Build history of the part. All positions in model axes, mm. Face numbers are marked on the shaded views. A direction names the side the tool comes from. Give positions to 0.01 mm unless a question says otherwise; leave off trailing zeros. Order: outer loops, then holes, each group sorted by start corner. A loop starts at its lowest first (then second) coordinate and runs counter-clockwise, first axis right, second up. Notation, with made-up numbers: (41, 30) -> (47, 30) arc R27 ccw to (47, 64) -> close; hole circle Ø4 at (-7.5, -34). An arc over 180 degrees is marked (long way). One line per item, written item: value. Start each with the question number.
(1) Probe line 1 (Y direction, x = -20.5, z = 8.5); line 2 (Z direction, x = -11, y = 18.5); line 3 (Y direction, x = 6.5, z = -9.5). List the from-to ranges inside material, lowest first.
(2) Saw through at C-C on y = 14.5. Give the cut face in (x, z).
(3) Saw through at D-D on x = 38. Give the cut face in (y, z).
(4) Two-plate mould, pull along Y, no slides. Class the marked faces 1, 2 and 3: +Y half, -Y half, draft (parallel to the pull), parting line (faces both ways), or undercut.
(5) Saw through at A-A on x = -11. Give the cut face in (y, z).
(6) Saw through at B-B on z = 13. Give the cut face in (x, y).
(7) Which spindle directions (+Z, -Z, +X, -X, +Y, -Y) get a long thin tool onto all of the face, cutting with end or side? Do the marked faces 4, 5 and 6. Say none if no direction does.
(8) Pin check, flat tips, straight feed: pin 1 (2.5 mm diameter, centred on y = 22, z = 4.5, fed in from -X); pin 2 (8 mm diameter, centred on x = -19, z = -1, fed in from +Y); pin 3 (15 mm diameter, centred on y = 13.5, z = 6.5, fed in from +X). Stop position of each tip, or through.
```python
from build123d import *

# Parameters (mm, degrees)
SKETCH1_W           = 90
SKETCH1_H           = 60
BOSS_EXTRUDE2_DEPTH = 25
CUT_EXTRUDE1_START  = 25
SKETCH2_W           = 45
SKETCH2_H           = 60
CUT_EXTRUDE1_DEPTH  = 5
SKETCH4_W           = 59
SKETCH4_H           = 24
CUT_EXTRUDE3_DEPTH  = 44.5
CUT_EXTRUDE4_START  = -45.5
SKETCH5_W           = 59
SKETCH5_H           = 19
CUT_EXTRUDE4_DEPTH  = 45


with BuildPart() as part:
    # Sketch1 → Boss-Extrude2 (new body)
    with BuildSketch(Plane(origin=(0, 0, 0), x_dir=(1, 0, 0), z_dir=(0, 1, 0))):
        with Locations((6.260188088, 2.087774295)):
            Rectangle(SKETCH1_W, SKETCH1_H)
    extrude(amount=BOSS_EXTRUDE2_DEPTH)

    # Sketch2 → Cut-Extrude1 (cut)
    with BuildSketch(Plane(origin=(0, 0, 0), x_dir=(1, 0, 0), z_dir=(0, 1, 0)).offset(CUT_EXTRUDE1_START)):
        with Locations((-16.239811912, 2.087774295)):
            Rectangle(SKETCH2_W, SKETCH2_H)
    extrude(amount=-CUT_EXTRUDE1_DEPTH, mode=Mode.SUBTRACT)

    # Sketch4 → Cut-Extrude3 (cut)
    with BuildSketch(Plane(origin=(51.260188088, 0, 0), x_dir=(0, 0, -1), z_dir=(1, 0, 0))):
        with Locations((2.087774295, 12.5)):
            Rectangle(SKETCH4_W, SKETCH4_H)
    extrude(amount=-CUT_EXTRUDE3_DEPTH, mode=Mode.SUBTRACT)

    # Sketch5 → Cut-Extrude4 (cut)
    with BuildSketch(Plane.ZY.offset(38.739811912).offset(CUT_EXTRUDE4_START)):
        with Locations((-2.087774295, 10)):
            Rectangle(SKETCH5_W, SKETCH5_H)
    extrude(amount=CUT_EXTRUDE4_DEPTH, mode=Mode.SUBTRACT)


solid = part.part
```
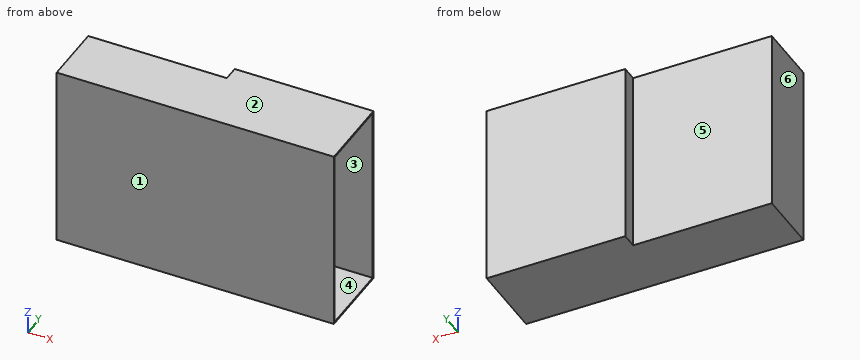
Results below:
1. line 1: y = 0 to 0.5, 19.5 to 20
1. line 2: z = -32.09 to -31.59, 27.41 to 27.91
1. line 3: y = 0 to 0.5, 19.5 to 25
2. outline: (-38.74, -32.09) -> (51.26, -32.09) -> (51.26, -31.59) -> (-38.24, -31.59) -> (-38.24, 27.41) -> (51.26, 27.41) -> (51.26, 27.91) -> (-38.74, 27.91) -> close
3. outline: (0, -32.09) -> (25, -32.09) -> (25, 27.91) -> (0, 27.91) -> close; hole (0.5, -31.59) -> (24.5, -31.59) -> (24.5, 27.41) -> (0.5, 27.41) -> close
4. face 1: -Y half
4. face 2: draft
4. face 3: undercut
5. outline: (0, -32.09) -> (20, -32.09) -> (20, 27.91) -> (0, 27.91) -> close; hole (0.5, -31.59) -> (19.5, -31.59) -> (19.5, 27.41) -> (0.5, 27.41) -> close
6. outline: (-38.74, 0) -> (51.26, 0) -> (51.26, 0.5) -> (-38.24, 0.5) -> (-38.24, 19.5) -> (6.76, 19.5) -> (6.76, 24.5) -> (51.26, 24.5) -> (51.26, 25) -> (6.26, 25) -> (6.26, 20) -> (-38.74, 20) -> close
7. face 4: +X
7. face 5: +Z, -Z, -X, +Y
7. face 6: +Z, -Z, -X, +Y, -Y
8. pin 1: stops at x = 6.26
8. pin 2: stops at y = 20
8. pin 3: stops at x = 6.76
